Study the drawing (mm; zero at the part's minimum x, y, z) and answer. Give positions to 0.01 mm unless a question says otherwise; leave off trailing zeros. Write each loop counter-clockwise with the first axis right and the second up, starting at its lowest first coordinate (ties: lowest second). Pieces come first, ordered by that corner, then holes. Notation, with made-up numbers: (11.25, -12) -> (51.25, -12) arc R22 ccw to (51.25, 0) -> close; hole circle Ø3 at (-14.5, -26). An arc over 180 degrees is marked (long way). Put each result on its own line as item: value. Start each with the question number.
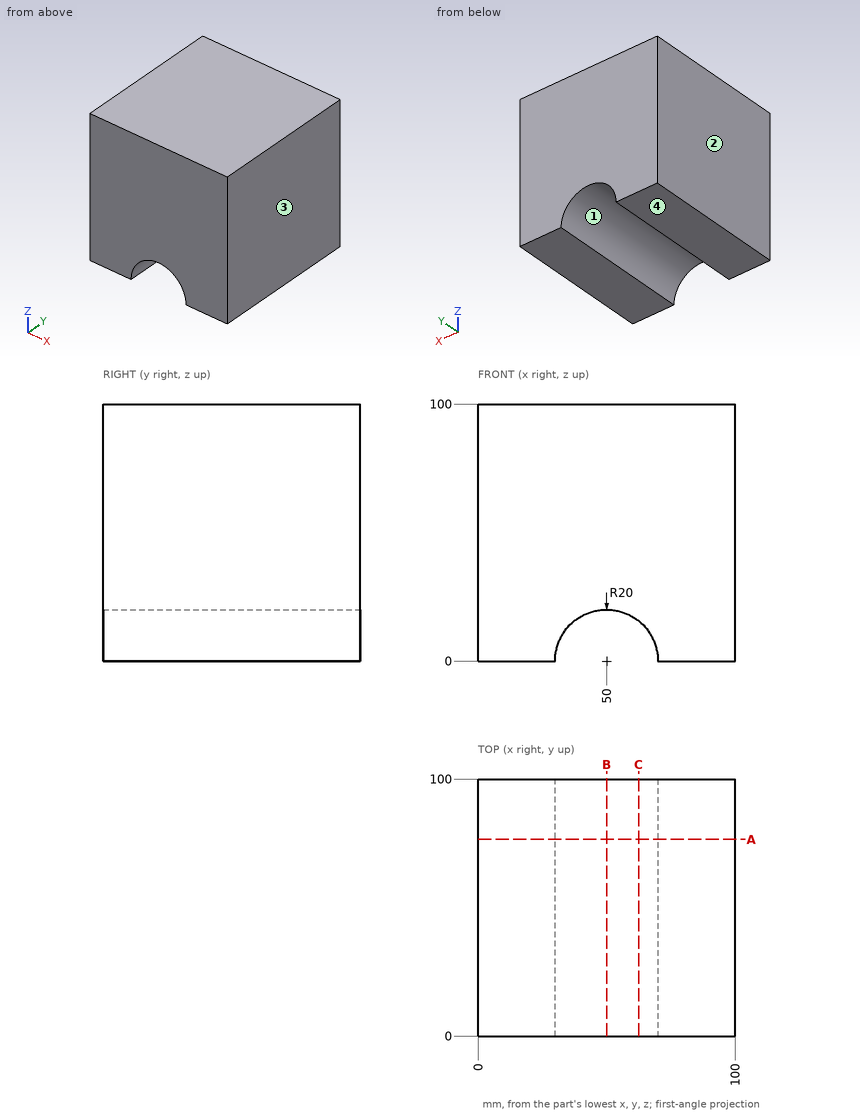
1) A cutting plane is placed at A-A on y = 76.5. Give the vertices of the cut face in (x, z).
2) For a pull along X with two mould halves and no side action, classify the marked faces 1, 2, 3 and 4 as pulls with the +X half, pulls with the -X half, needs draft (parallel to the pull), parting line crosses it, or undercut.
3) Straight lines are drawn through the part: line 1 (X direction, y = 21.5, z = 17); line 2 (X direction, y = 28, z = 16); line 3 (Z direction, x = 61, y = 76.5). For each, find the intervals that lie inside material, in ascending order. Write a range as [from, to].
4) A cutting plane is placed at B-B on x = 50. Give the vertices of the cut face in (y, z), and give its area (3 significant figures).
5) A cutting plane is placed at C-C on x = 62.5. Give the vertices of the cut face in (y, z), and give its area (3 significant figures).
Results found:
1. outline: (0, 0) -> (30, 0) arc R20 cw to (70, 0) -> (100, 0) -> (100, 100) -> (0, 100) -> close
2. face 1: undercut
2. face 2: pulls with the -X half
2. face 3: pulls with the +X half
2. face 4: needs draft
3. line 1: x = [0, 39.46], [60.54, 100]
3. line 2: x = [0, 38], [62, 100]
3. line 3: z = [16.7, 100]
4. outline: (0, 20) -> (100, 20) -> (100, 100) -> (0, 100) -> close
4. area: 8,000 mm²
5. outline: (0, 15.61) -> (100, 15.61) -> (100, 100) -> (0, 100) -> close
5. area: 8,440 mm²
